```python
from build123d import *

# Parameters (mm, degrees)
BOSS_EXTRUDE1_DEPTH = 3.302
SHELL3_T            = -1.016
FILLET2_R           = 2.54


with BuildPart() as part:
    # Sketch1 → Boss-Extrude1 (new body)
    with BuildSketch(Plane(origin=(0, 0, 0), x_dir=(1, 0, 0), z_dir=(0, 1, 0))):
        with BuildLine():
            Line((0, 0), (65.786, 0))
            ThreePointArc((65.786, 0), (74.93, -9.144), (65.786, -18.288))
            Line((65.786, -18.288), (25.4, -18.288))
            Line((25.4, -18.288), (23.114, -14.224))
            Line((23.114, -14.224), (-14.224, -14.224))
            ThreePointArc((-14.224, -14.224), (-10.057886856, -4.166113144), (0, 0))
        make_face()
    extrude(amount=BOSS_EXTRUDE1_DEPTH)

    # Shell3
    shell3_openings = [part.faces().sort_by_distance(p)[0] for p in [
        (28.676685524, 3.302, 10.346352191),
    ]]
    offset(amount=SHELL3_T, openings=shell3_openings, kind=Kind.INTERSECTION)

    # Fillet2
    fillet2_edges = [part.edges().sort_by_distance(p)[0] for p in [
        (32.893, 0, 0),
        (74.93, 0, 9.144),
        (45.593, 0, 18.288),
        (24.257, 0, 16.256),
        (4.445, 0, 14.224),
        (-10.057886856, 0, 4.166113144),
    ]]
    fillet(fillet2_edges, radius=FILLET2_R)


solid = part.part
```
Source: CAD feature listing. Evaluate the final solid. Frame: model axes, mm. A direction names the side the tool comes from. Round coordinates to 2 decimals unless told otherwise and drop trailing zeros. Loops run counter-clockwise (first coordinate to the right, second up) from the corner with the lowest first, then second, coordinate; pieces in that order, holes last.
1. Mould query, pull axis X, two halves, no side actions, for faces 4 (the flat face through (40, 0, 9)), 5 (the cylindrical face through (74.928, 2.916, 8.943)), 6 (the flat face through (31, 1.016, 9)). Classes: released by +X, released by -X, zero draft, split by the parting line, or undercut.
2. Section query A-A on y = 2. Output: boundary loops of the cut face in (x, z).
3. Access query for faces 1 (the flat face through (33.9, 3.302, 0.3)), 2 (the cylindrical face through (73.912, 2.143, 8.965)), 3 (the cylindrical face through (4.916, 0.764, 13.5)). Directions: +Z, -Z, +X, -X, +Y, -Y. A direction counts if a zero-diameter tool reaches every point of the face in a straight line with its end or side. Return the directions, or none.
4. Section query C-C on x = 37.5. Output: boundary loops of the cut face in (y, z), and give its area (3 significant figures).
5. Section query B-B on x = 8. Output: boundary loops of the cut face in (y, z).
6. Ray query, L1, parallel to Z at x = 55.5, y = 2.5; L2, parallel to Y at x = 29, z = 10.75; L3, parallel to Z at x = 22.5, y = 1.95. Return the intervals inside material, ascending.
7. Contact query for flat-ended pins moving along their axis: pin 1 (1.1 mm diameter, centred on x = 23.5, y = 2, fed in from +Z); pin 2 (0.7 mm diameter, centred on x = 38, y = 2, fed in from -Z); pin 3 (1 mm diameter, centred on x = 38.5, z = 10, fed in from +Y). Output: stop coordinate, or through.
Answers below:
1. face 4: zero draft
1. face 5: released by +X
1. face 6: undercut
2. outline: (-14.17, 14.17) arc R14.17 ccw to (0, 0.06) - (65.79, 0.06) arc R9.09 ccw to (65.79, 18.23) - (25.43, 18.23) - (23.15, 14.17) - close; hole (-13.17, 13.21) arc R13.21 ccw to (0, 1.02) - (65.79, 1.02) arc R8.13 ccw to (65.79, 17.27) - (25.99, 17.27) - (23.71, 13.21) - close
3. face 1: +Z, -Z, +X, -X, +Y
3. face 2: +Y
3. face 3: +Z, -X, -Y
4. outline: (0, 2.54) arc R2.54 ccw to (2.54, 0) - (3.3, 0) - (3.3, 1.02) - (1.02, 1.02) - (1.02, 17.27) - (3.3, 17.27) - (3.3, 18.29) - (2.54, 18.29) arc R2.54 ccw to (0, 15.75) - close
4. area: 20.5 mm2
5. outline: (0, 2.54) arc R2.54 ccw to (2.54, 0) - (3.3, 0) - (3.3, 1.02) - (1.02, 1.02) - (1.02, 13.21) - (3.3, 13.21) - (3.3, 14.22) - (2.54, 14.22) arc R2.54 ccw to (0, 11.68) - close
6. L1: z = 0 to 1.02, 17.27 to 18.29
6. L2: y = 0 to 1.02
6. L3: z = 0.07 to 1.02, 13.21 to 14.15
7. pin 1: stops at z = 15.79
7. pin 2: stops at z = 0.01
7. pin 3: stops at y = 1.02
